The model under review builds one solid part; all positions refer to its coordinate system, in mm. Face numbers are marked on the shaded views. A direction names the side the tool comes from. Round coordinates to 2 decimals unless told otherwise and drop trailing zeros. Order: outer loops, then holes, each group sorted by start corner. A loop starts at its lowest first (then second) coordinate and runs counter-clockwise, first axis right, second up.
1) Consider section B-B (z = 4). Give the boundary of the cut face in (x, y).
2) Consider section D-D (x = 10.5). Give the boundary of the cut face in (y, z), then the cut area to 3 significant figures.
3) Mouldability with a two-part tool opening along X and no side actions: class the marked faces 3, 4, 5 and 6 as pulls with the +X half, pulls with the -X half, needs draft (parallel to the pull), parting line crosses it, or undercut.
4) Consider section A-A (y = 7). Give the boundary of the cut face in (x, z) (1 decimal), then the cut area to 3 significant figures.
5) Consider section C-C (x = 0). Give the boundary of the cut face in (y, z).
6) To check wall thickness, follow L1, parallel to Z at x = 6, y = 8.25; L2, parallel to Z at x = -2, y = 3.25; L3, parallel to X at y = 0.75, z = 4. State the ranges of each line that lie inside material, in increasing order.
7) Clearance check with flat-ended pins moving along their axes: P1, Ø1.5, axis at x = 14.5, y = 8, coming from the +Z side; P2, Ø2, axis at x = -3.5, y = 1.5, coming from the +Z side; P3, Ø5, axis at y = 4, z = -3.5, coming from the +X side. State where each tip first meets the part, or that it passes through.
8) Machinability: for the marked faces 1 and 2, which of the approach directions +Z, -Z, +X, -X, +Y, -Y give a long, thin tool a straight path to every point of the face, cutting with its end or side? Answer none if there is none.
from build123d import *

# Parameters (mm, degrees)
SKETCH1_R           = 30.1625
BOSS_EXTRUDE1_DEPTH = 10.16
CUT_EXTRUDE1_DEPTH  = 11.16
SKETCH3_R           = 30.1625
SKETCH3_R_2         = 23.8125
CUT_EXTRUDE2_DEPTH  = 11.16


with BuildPart() as part:
    # Sketch1 → Boss-Extrude1 (new body)
    with BuildSketch(Plane(origin=(0, 0, 0), x_dir=(1, 0, 0), z_dir=(0, 1, 0))):
        Circle(SKETCH1_R)
    extrude(amount=BOSS_EXTRUDE1_DEPTH)

    # Sketch2 → Cut-Extrude1 (cut, through all)
    with BuildSketch(Plane(origin=(0, 10.16, 0), x_dir=(1, 0, 0), z_dir=(0, 1, 0))):
        Polygon((4.067255107, -6.10088266), (7.317146922, 0.471904916), (3.249891816, 6.572787576), (-4.067255107, 6.10088266), (-7.317146922, -0.471904916), (-3.249891816, -6.572787576), align=None)
    extrude(amount=-CUT_EXTRUDE1_DEPTH, mode=Mode.SUBTRACT)

    # Sketch3 → Cut-Extrude2 (cut, through all)
    with BuildSketch(Plane(origin=(0, 0, 0), x_dir=(-1, 0, 0), z_dir=(0, -1, 0))):
        Circle(SKETCH3_R)
        Circle(SKETCH3_R_2, mode=Mode.SUBTRACT)
    extrude(amount=-CUT_EXTRUDE2_DEPTH, mode=Mode.SUBTRACT)


solid = part.part
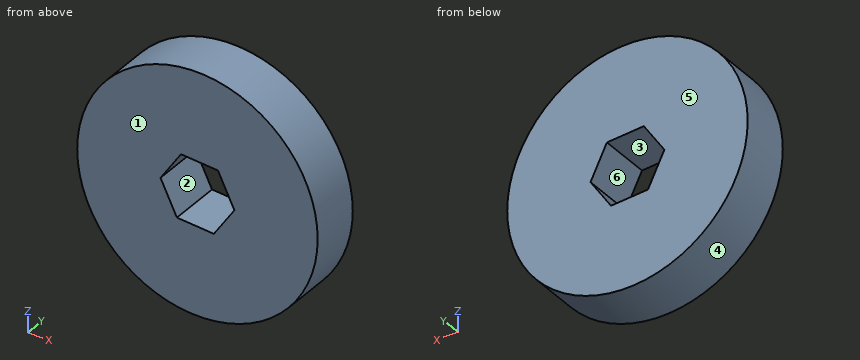
Answer below:
1. outline: (-23.47, 0) - (-4.97, 0) - (-4.97, 10.16) - (-23.47, 10.16) - close; (5.11, 0) - (23.47, 0) - (23.47, 10.16) - (5.11, 10.16) - close
2. outline: (0, -21.37) - (10.16, -21.37) - (10.16, 21.37) - (0, 21.37) - close
2. area: 434 mm2
3. face 3: undercut
3. face 4: parting line crosses it
3. face 5: needs draft
3. face 6: undercut
4. outline: circle Ø47.6 at (0, 0); hole (-7.3, 0.5) - (-4.1, -6.1) - (3.2, -6.6) - (7.3, -0.5) - (4.1, 6.1) - (-3.2, 6.6) - close
4. area: 1,640 mm2
5. outline: (0, -23.81) - (10.16, -23.81) - (10.16, -6.36) - (0, -6.36) - close; (0, 6.36) - (10.16, 6.36) - (10.16, 23.81) - (0, 23.81) - close
6. L1: z = -23.04 to -2.45, 2.19 to 23.04
6. L2: z = -23.73 to -6.23, 6.49 to 23.73
6. L3: x = -23.47 to -4.97, 5.11 to 23.47
7. P1: stops at z = 19.44
7. P2: stops at z = 23.68
7. P3: stops at x = 23.79
8. face 1: +Z, -Z, +X, -X, -Y
8. face 2: +Y, -Y
